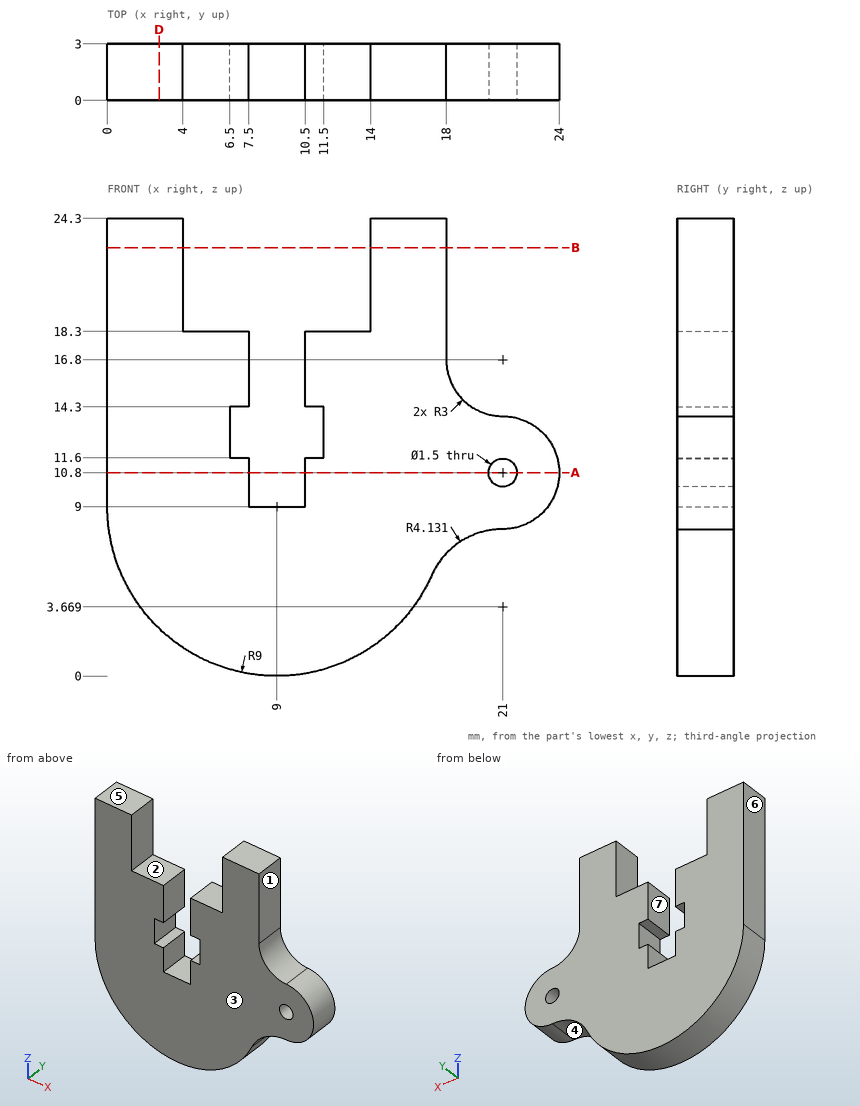
For this review, use the dimensioned drawing (mm, ordinates from the lowest corner) and the shaded views. A direction names the side the tool comes from. Give positions to 0.01 mm unless a question says otherwise; leave off trailing zeros. Loops run counter-clockwise (first coordinate to the right, second up) from the corner with the lowest first, then second, coordinate; pieces in that order, holes last. Notation, with made-up numbers: (-5.5, 15.5) -> (36.5, 15.5) arc R5 cw to (36.5, 21.5) -> close; hole circle Ø11 at (69, 6.5). An arc over 180 degrees is marked (long way). Use CSV: the item, a comma, the result in double quotes.
1. Machinability: for the marked faces 1, 2 and 3, which of the approach directions +Z, -Z, +X, -X, +Y, -Y give a long, thin tool a straight path to every point of the face, cutting with its end or side? Answer none if there is none.
Result:
face 1,"+Z, +X, +Y, -Y"
face 2,"+Z, +Y, -Y"
face 3,"+Z, -Z, +X, -X, -Y"
2. Consider section A-A, the plane z = 10.8. Write out the cut boundary in (x, y), then the cut area to 3 significant figures.
Result:
outline,"(0, 0) -> (7.5, 0) -> (7.5, 3) -> (0, 3) -> close; (10.5, 0) -> (20.25, 0) -> (20.25, 3) -> (10.5, 3) -> close; (21.75, 0) -> (24, 0) -> (24, 3) -> (21.75, 3) -> close"
area,"58.5 mm²"
3. Consider section B-B, the plane z = 22.75. Write out the cut boundary in (x, y), then the cut area to 3 significant figures.
Result:
outline,"(0, 0) -> (4, 0) -> (4, 3) -> (0, 3) -> close; (14, 0) -> (18, 0) -> (18, 3) -> (14, 3) -> close"
area,"24.0 mm²"
4. To check wall thickness, follow probe 1 along X at (y, z) = (1.5, 10.8); probe 2 along X at (y, z) = (2.8, 21); probe 3 along Z at (x, y) = (6.75, 0.7). State the ranges of each line that lie inside material, in increasing order. Write a range as from..to.
Result:
probe 1,"x = 0..7.5, 10.5..20.25, 21.75..24"
probe 2,"x = 0..4, 14..18"
probe 3,"z = 0.29..11.6, 14.3..18.3"
5. The part is to be moulded in two halves that separate along X. For the marked faces 4, 5, 6 and 7, say which applies: +X half, -X half, draft (parallel to the pull), parting line (faces both ways), or undercut.
Result:
face 4,"+X half"
face 5,"draft"
face 6,"-X half"
face 7,"undercut"
6. Consider section D-D, the plane x = 2.75. Write out the cut boundary in (y, z).
Result:
outline,"(0, 2.52) -> (3, 2.52) -> (3, 24.3) -> (0, 24.3) -> close"
7. For P1, Ø0.9, axis at y = 1, z = 16.5, coming from the +X side (1 decimal); P2, Ø0.9, axis at x = 5.5, y = 1.5, coming from the +Z side; P3, Ø1.5, axis at y = 1.5, z = 21, coming from the +X side; P4, Ø0.9, axis at x = 21, z = 10.8, coming from the +Y side, all flat-tipped, find the tip position at first contact; note any pin that passes through.
Result:
P1,"stops at x = 18.1"
P2,"stops at z = 18.3"
P3,"stops at x = 18"
P4,"passes through"
